CAD build for the part. Positions are in the model's coordinates, mm. A direction names the side the tool comes from. Give positions to 0.01 mm unless a question says otherwise; leave off trailing zeros. Order: outer loops, then holes, each group sorted by start corner. A loop starts at its lowest first (then second) coordinate and runs counter-clockwise, first axis right, second up. Notation, with made-up numbers: (-9.75, 86.25) -> (26.25, 86.25) arc R20 ccw to (26.25, 103.25) -> close; hole circle Ø3 at (-12.75, 19.25). An arc over 180 degrees is marked (long way). Use one line per item in the form item = value. Start each with the question number.
1) Cut at A-A, the plane z = 10. Give the cut face in (x, y), and give its area (3 significant figures).
2) Cut at C-C, the plane z = 1.75. Give the cut face in (x, y).
3) Cut at D-D, the plane y = -31.5. Give the cut face in (x, z), and give its area (3 significant figures).
4) Probe line 1 (X direction, y = -35, z = 10); line 2 (X direction, y = -33.5, z = 9.75); line 3 (Y direction, x = 19, z = 4.75). List the from-to ranges inside material, lowest first.
5) Tool access for faces 1 (the face through (19, -39.765, 10)), 2 (the face through (18.604, -17.573, 9.86)), 3 (the face through (2.95, -35.33, 11.25)): list every direction of +Z, -Z, +X, -X, +Y, -Y with a clear straight run to the whole face (end or side of a thin tool).
6) Mould opens along Z. For faces 4 (the face through (14.4, -35.33, 5.23)), 5 (the face through (7.024, -17.938, 9.86)), 6 (the face through (8, -13, 20)) say: pulls with the +Z half, pulls with the -Z half, needs draft (parallel to the pull), parting line crosses it, or undercut.
7) Cut at B-B, the plane y = -25.5. Give the cut face in (x, z).
8) Drop flat-ended pins along their axis: P1, Ø2, axis at x = 20.5, z = 11.5, coming from the +Y side; P2, Ø1.5, axis at x = 22.9, z = 10, coming from the +Y side; P3, Ø8, axis at y = -5, z = 7.5, coming from the +X side. Give the stop position or say it passes through.
from build123d import *

# Parameters (mm, degrees)
SALIENTE_EXTRUIR1_DEPTH = 20
CROQUIS4_R              = 5
CROQUIS4_R_2            = 1.25
CORTAR_EXTRUIR3_DEPTH   = 9


with BuildPart() as part:
    # Croquis1 → Saliente-Extruir1 (new body)
    with BuildSketch(Plane.XY):
        with BuildLine():
            Line((-12.104887717, -39.764697086), (7.777460826, 0))
            ThreePointArc((7.777460826, 0), (12.895112283, 12.355103555), (18.01276374, 0))
            Line((18.01276374, 0), (37.895112283, -39.764697086))
            Line((37.895112283, -39.764697086), (-12.104887717, -39.764697086))
        make_face()
        Polygon((1.314448857, -30.764697086), (12.895112283, -4.746347114), (24.475775709, -30.764697086), (14.62955151, -30.764697086), align=None, mode=Mode.SUBTRACT)
    extrude(amount=SALIENTE_EXTRUIR1_DEPTH)

    # Croquis4 → Cortar-Extruir3 (cut)
    with BuildSketch(Plane.XZ.offset(39.764697086)):
        with Locations(Location((12.895112283, 10, 0), (0, 0, 270))):
            Circle(CROQUIS4_R)
        with Locations(Location((22.895112283, 10, 0), (0, 0, 270))):
            Circle(CROQUIS4_R_2)
        with Locations(Location((2.895112283, 10, 0), (0, 0, 270))):
            Circle(CROQUIS4_R_2)
    extrude(amount=-CORTAR_EXTRUIR3_DEPTH, mode=Mode.SUBTRACT)


solid = part.part
Result:
q1.outline = (-12.1, -39.76) -> (1.65, -39.76) -> (1.65, -30.76) -> (1.31, -30.76) -> (12.9, -4.75) -> (24.48, -30.76) -> (24.15, -30.76) -> (24.15, -39.76) -> (37.9, -39.76) -> (18.01, 0) arc R7.24 ccw (long way) to (7.78, 0) -> close; (4.15, -39.76) -> (7.9, -39.76) -> (7.9, -30.76) -> (4.15, -30.76) -> close; (17.9, -39.76) -> (21.65, -39.76) -> (21.65, -30.76) -> (17.9, -30.76) -> close
q1.area = 911 mm²
q2.outline = (-12.1, -39.76) -> (37.9, -39.76) -> (18.01, 0) arc R7.24 ccw (long way) to (7.78, 0) -> close; hole (1.31, -30.76) -> (24.48, -30.76) -> (12.9, -4.75) -> close
q3.outline = (-7.97, 0) -> (33.76, 0) -> (33.76, 20) -> (-7.97, 20) -> close; hole circle Ø2.5 at (2.9, 10); hole circle Ø10 at (12.9, 10); hole circle Ø2.5 at (22.9, 10)
q3.area = 746 mm²
q4.line_1 = -9.72 to 1.65, 4.15 to 7.9, 17.9 to 21.65, 24.15 to 35.51
q4.line_2 = -8.97 to 1.67, 4.12 to 7.9, 17.89 to 21.67, 24.12 to 34.76
q4.line_3 = -39.76 to -30.76, -18.46 to -1.97, 1.23 to 9
q5.face_1 = +Z, -Z, +X, -X, -Y
q5.face_2 = +Z, -Z
q5.face_3 = -Y
q6.face_4 = undercut
q6.face_5 = needs draft
q6.face_6 = pulls with the +Z half
q7.outline = (-4.97, 0) -> (3.66, 0) -> (3.66, 20) -> (-4.97, 20) -> close; (22.13, 0) -> (30.76, 0) -> (30.76, 20) -> (22.13, 20) -> close
q8.P1 = 8.08
q8.P2 = -8.27
q8.P3 = 22.51
